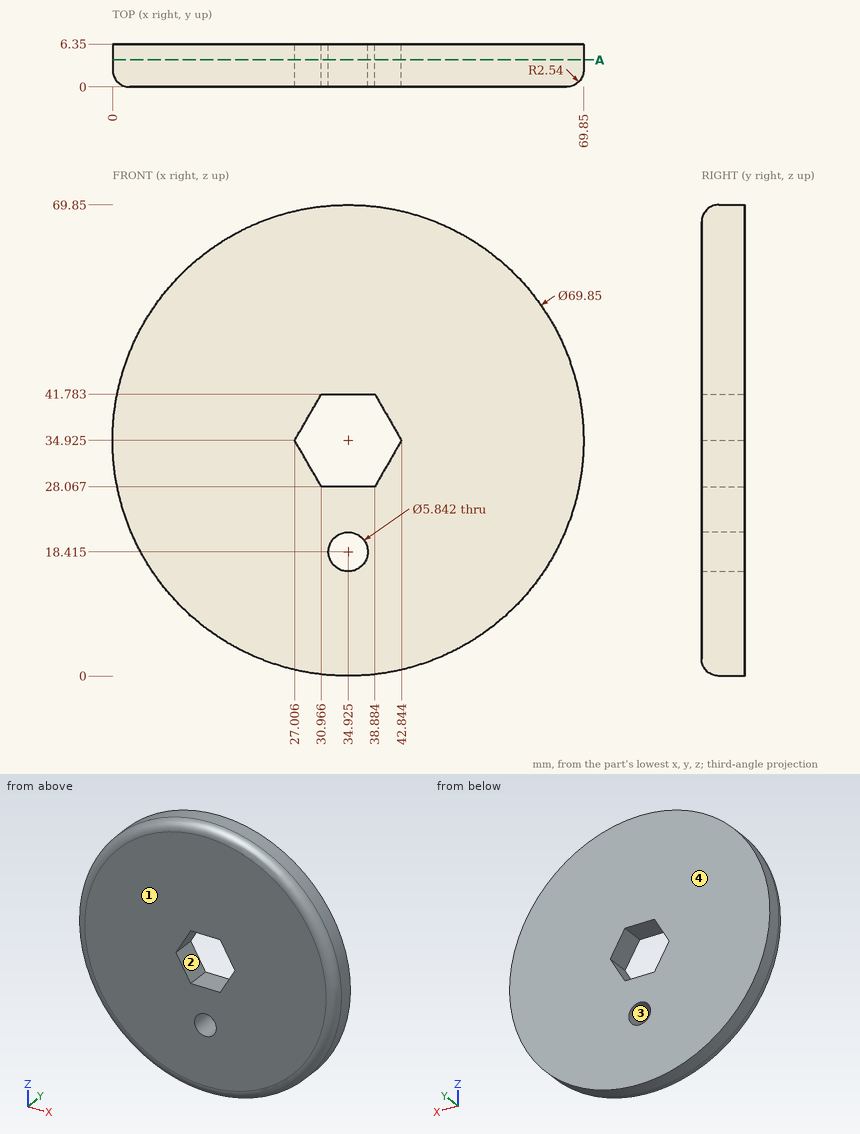
Verification items for this drawing (mm, ordinates from the low corner). A direction names the side the tool comes from. Coordinates: 2 decimals unless noted, no trailing zeros. Answer as a JSON object with one key per item and string values. Group by question number.
(1) Gauge pin test, flat ends, axial feed: pin 1 (2 mm diameter, centred on x = 37.5, y = 5, fed in from -Z) (1 decimal); pin 2 (1.5 mm diameter, centred on x = 13, y = 5.5, fed in from -Z); pin 3 (2 mm diameter, centred on y = 2.5, z = 34.5, fed in from +X). Record the tip position at first contact, or that the pin passes through.
(2) Cross-section at A-A, the plane y = 4. State how many separate pieces and enclosed holes the cut face has, and give its area (3 significant figures).
(3) Tool access check on the marked faces 1 and 2. Record the directions out of +Z, -Z, +X, -X, +Y, -Y that give a thin tool (end or side, any length) a straight path to the whole face; none if there is none.
(4) Material ranges on line 1 (Z direction, x = 33, y = 2.25) (1 decimal); line 2 (X direction, y = 6, z = 39); line 3 (X direction, y = 3.75, z = 16.5) (1 decimal), recorded low to high.
(5) Release check for a two-part mould opening along X. For the marked faces 3 and 4 record: +X half, -X half, draft (parallel to the pull), parting line (faces both ways), or undercut.
Reply:
{
 "1": {"pin 1": "z = 0", "pin 2": "z = 7.15", "pin 3": "x = 69.85"},
 "2": {"separate pieces": "1", "enclosed holes": "2", "area": "3,640 mm²"},
 "3": {"face 1": "+Z, -Z, +X, -X, -Y", "face 2": "+Y, -Y"},
 "4": {"line 1": "0.1 to 16.2, 20.6 to 28.1, 41.8 to 69.8", "line 2": "0.24 to 29.36, 40.49 to 69.61", "line 3": "5.3 to 32.7, 37.1 to 64.6"},
 "5": {"face 3": "undercut", "face 4": "draft"}
}
